from build123d import *

# Parameters (mm, degrees)
F2_SIZE = 5


with BuildPart() as f1:
    # F0 (on Front) → F1 (revolve)
    with BuildSketch(Plane.XZ):
        Polygon((-40, -20), (-40, 0), (-50.75, 0), (-50.75, -25.5), (-63, -25.5), (-63, -35.5), (-45, -35.5), (-45, -56), (-35.5, -56), (-35.5, -41), (-33, -41), (-33, -25), (-36, -25), (-36, -20), align=None)
    revolve(axis=Axis((0, 0, -28), (0, 0, -1)))

    # F2
    f2_edges = [f1.edges().sort_by_distance(p)[0] for p in [
        (63, 0, -35.5),
        (45, 0, -35.5),
    ]]
    chamfer(f2_edges, length=F2_SIZE)


solid = f1.part
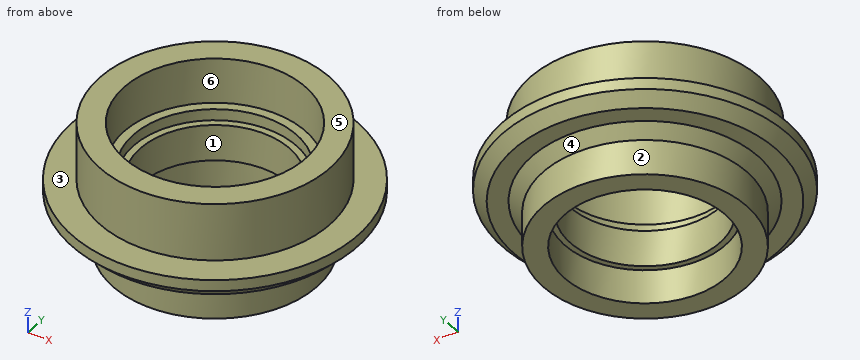
CAD build for the part. Positions are in the model's coordinates, mm. Face numbers are marked on the shaded views. A direction names the side the tool comes from. Coordinates: 2 decimals unless noted, no trailing zeros. Order: outer loops, then holes, each group sorted by start corner. A loop starts at its lowest first (then second) coordinate and runs counter-clockwise, first axis right, second up.
Item 1: Band-saw the part on D-D on z = -21.5. List the corners of the cut face in (x, y), plus the area to 3 significant figures.
Check sheet entries:
outline: circle Ø101.5 at (0, 0); hole circle Ø72 at (0, 0)
area: 4,020 mm2
Item 2: Two-plate mould, pull along X, no slides. Class the marked faces 4, 5 and 6: +X half, -X half, draft (parallel to the pull), parting line (faces both ways), or undercut.
Check sheet entries:
face 4: parting line
face 5: draft
face 6: undercut
Item 3: Drill centre lines: L1, parallel to Y at x = 0, z = -10.75; L2, parallel to Y at x = 0, z = -23.8; L3, parallel to Z at x = 36, y = -2. Where is each one in solid material? Low to high.
Check sheet entries:
L1: y = -50.75 to -40, 40 to 50.75
L2: y = -50.75 to -36, 36 to 50.75
L3: z = -56 to -20
Item 4: 3-axis set-ups, long thin cutter, end or side, ignore diameter. For the marked faces 1, 2 and 3: which of +Z, -Z, +X, -X, +Y, -Y reach the whole face in a straight line?
Check sheet entries:
face 1: +Z, -Z
face 2: -Z
face 3: +Z
Item 5: Band-saw the part on C-C on z = -43.5. List the corners of the cut face in (x, y).
Check sheet entries:
outline: circle Ø90 at (0, 0); hole circle Ø71 at (0, 0)
Item 6: Pin check, flat tips, straight feed: pin 1 Ø1 at (y, z) = (20, -20) entering from +X; pin 2 Ø10 at (x, y) = (6.5, -28.5) entering from +Z; pin 3 Ø12 at (x, z) = (-43, -16) entering from -Y. Stop position of each tip, or through.
Check sheet entries:
pin 1: stops at x = 46.85
pin 2: stops at z = -25
pin 3: stops at y = -34.74
